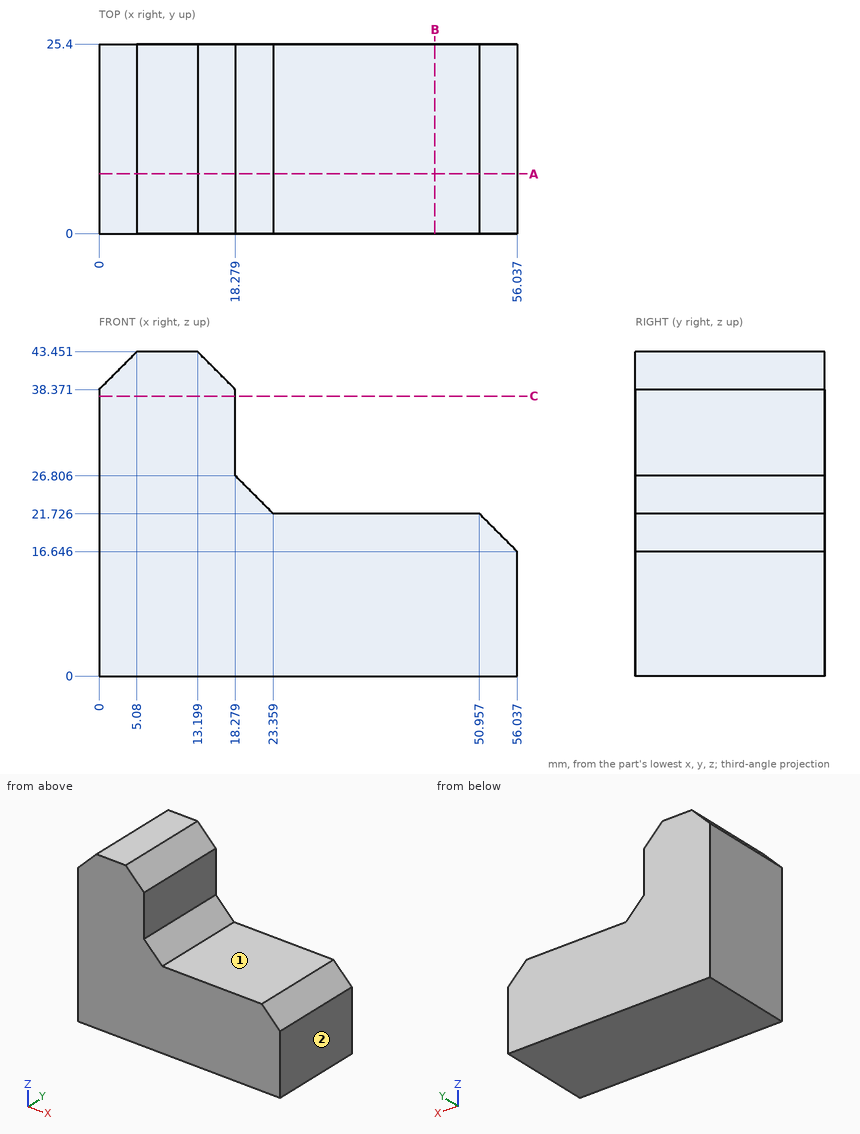
Input: dimensioned drawing with shaded views. Units: mm. Origin: part minimum x, y, z. A direction names the side the tool comes from. Round coordinates to 2 decimals unless told otherwise and drop trailing zeros. Loops run counter-clockwise (first coordinate to the right, second up) from the corner with the lowest first, then second, coordinate; pieces in that order, holes last. Notation, with made-up numbers: M -37.75,-28.5 L -6.75,-28.5 A16 ccw -6.75,-22.5 Z; hole C -2.5,88 d4. An arc over 180 degrees is marked long. One line per question, with ' | ' between items.
(1) Contact query for flat-ended pins moving along their axis: P1, Ø5, axis at x = 29, y = 6, coming from the +Z side; P2, Ø6, axis at y = 18.5, z = 34, coming from the +X side. Output: stop coordinate, or through.
Check result:
P1: stops at z = 21.73 | P2: stops at x = 18.28
(2) Cut plane C-C on z = 37.5. Return the cut outline in (x, y), plus the area to 3 significant figures.
Check result:
outline: M 0,0 L 18.28,0 L 18.28,25.4 L 0,25.4 Z | area: 464 mm2
(3) Cut plane B-B on x = 45. Return the cut outline in (y, z) (1 decimal), plus the area to 3 significant figures.
Check result:
outline: M 0,0 L 25.4,0 L 25.4,21.7 L 0,21.7 Z | area: 552 mm2
(4) Access query for the marked faces 1 and 2. Directions: +Z, -Z, +X, -X, +Y, -Y. A direction counts if a zero-diameter tool reaches every point of the face in a straight line with its end or side. Return the directions, or none.
Check result:
face 1: +Z, +X, +Y, -Y | face 2: +Z, -Z, +X, +Y, -Y
(5) Cut plane A-A on y = 8. Return the cut outline in (x, z) (1 decimal).
Check result:
outline: M 0,0 L 56,0 L 56,16.6 L 51,21.7 L 23.4,21.7 L 18.3,26.8 L 18.3,38.4 L 13.2,43.5 L 5.1,43.5 L 0,38.4 Z
(6) Material intervals for line 1 along Z through (x, y) = (45.5, 10.5) (1 decimal); line 2 along X through (y, z) = (22.5, 34); line 3 along X through (y, z) = (14.25, 24) (1 decimal), sorted ascending. Write a range as from..to.
Check result:
line 1: z = 0..21.7 | line 2: x = 0..18.28 | line 3: x = 0..21.1
